Check sheet for the modelled part. Datum: model origin and axes. Units: mm. A direction names the side the tool comes from. Coordinates: 2 decimals unless noted, no trailing zeros. Loops run counter-clockwise (first coordinate to the right, second up) from the corner with the lowest first, then second, coordinate; pieces in that order, holes last. Notation, with made-up numbers: (30, -6.75) - (63, -6.75) arc R17 ccw to (63, 20.25) - close; hole circle Ø6 at (-8.75, 21). An arc over 180 degrees is marked (long way). Use a Markdown table: item, result. Add a question column.
1) Tool access check on faces 4 (the flat face through (4.144, 2.348, -9.615)), 5 (the flat face through (-4.11, 2.41, -22.75)), 6 (the flat face through (0, 4.762, -10)), 7 (the flat face through (7, 0, 26.683)), 8 (the cylindrical face through (-1.09, -4.91, 5.2)). Record the directions out of +Z, -Z, +X, -X, +Y, -Y that give a thin tool (end or side, any length) a straight path to the whole face; none if there is none.
2) Go/stop test with flat-tipped pins: P1, Ø3, axis at x = -5, y = -2, coming from the -Z side; P2, Ø4.5, axis at x = -0.5, z = -6, coming from the +Y side; P3, Ø3, axis at y = -3, z = -8.5, coming from the +X side; P4, Ø6, axis at x = 1, z = -21, coming from the -Y side. Record where each tip stops, or that it passes through.
3) Sectioned sample at A-A, the plane y = 5.75. Enter the section's corners in (x, z).
4) Sectioned sample at C-C, the plane z = 18. Enter the section's corners in (x, y).
5) Thickness scan on line 1 (Z direction, x = 2, y = -5.25); line 2 (Z direction, x = -3.5, y = -3); line 3 (Y direction, x = 1.75, z = -3). Record the ranges inside material, lowest first.
6) Draft check along Z on faces 1 (the flat face through (0, 0, 33.668)), 2 (the cylindrical face through (-0.834, 3.757, -18.219)), 3 (the flat face through (0, -6.375, 2)). Enter one of: pulls with the +Z half, pulls with the -Z half, needs draft (parallel to the pull), parting line crosses it, or undercut.
7) Sectioned sample at B-B, the plane z = -23.5. Enter the section's corners in (x, y), then the cut area to 3 significant figures.
Autodesk Inventor part; units mm, degrees
ref_plane "Work Plane1" through (0, 0, 15.2527) normal (0, 0, 1) x (1, 0, 0)
ref_plane "Work Plane2" through (0, 0, 5.7785) normal (0, 0, 1) x (1, 0, 0)
ref_plane "Work Plane3" through (0, 0, -18.7071) normal (0, 0, 1) x (1, 0, 0)
sketch "Sketch1" plane through (0, 0, 0) normal (0, 0, 1) x (1, 0, 0)
  line L0 (-10.3063, 0) -> (10.3063, 0)
  line L1 (0, -8.9256) -> (0, 8.9256)
  line L2 (3.6808, 6.3754) -> (7.3617, 0)
  line L3 (7.3617, 0) -> (3.6808, -6.3754)
  line L4 (3.6808, -6.3754) -> (-3.6808, -6.3754)
  line L5 (-3.6808, -6.3754) -> (-7.3617, 0)
  line L6 (-7.3617, 0) -> (-3.6808, 6.3754)
  line L7 (-3.6808, 6.3754) -> (3.6808, 6.3754)
  point P0 (0, 0)
  point P1 (0, 0)
  point P2 (0, 6.3754)
  dimension "d0" = 12.7508
extrude "Base" add sketch "Sketch1" along normal mid plane 67.3354
sketch "Sketch2" plane through (0, 0, 33.6677) normal (0, 0, 1) x (1, 0, 0)
  line L0 (7.3617, 0) -> (3.6808, -6.3754)
  line L1 (3.6808, 6.3754) -> (7.3617, 0)
  line L2 (-3.6808, 6.3754) -> (3.6808, 6.3754)
  line L3 (-7.3617, 0) -> (-3.6808, 6.3754)
  line L4 (-3.6808, -6.3754) -> (-7.3617, 0)
  line L5 (3.6808, -6.3754) -> (-3.6808, -6.3754)
  circle A0 centre (0, 0) radius 6.3754
extrude "Bearing Fit" cut sketch "Sketch2" against normal blind 6.985 contours L0 A0 L1 | L0 L5 A0 | A0 L2 L1 | L5 L4 A0 | A0 L3 L2 | L4 L3 A0
mirror "Mirror1" about plane through (0, 0, 0) normal (0, 0, 1) of "Bearing Fit"
sketch "Sketch4" plane through (0, 0, -33.6677) normal (0, 0, -1) x (-1, 0, 0)
  circle A0 centre (0, 0) radius 6.3754
  circle A1 centre (0, 0) radius 4.7625
  dimension "d7" = 9.525
extrude "Extrusion4" cut sketch "Sketch4" against normal up to surface (6.985 mm away)
sketch "Sketch5" plane through (3.6808, 6.3754, -26.6827) normal (0, 0, -1) x (-1, 0, 0)
  line L0 (7.3617, 0) -> (11.0425, -6.3754)
  line L1 (0, 0) -> (7.3617, 0)
  line L2 (-3.6808, -6.3754) -> (0, 0)
  line L3 (0, -12.7508) -> (-3.6808, -6.3754)
  line L4 (7.3617, -12.7508) -> (0, -12.7508)
  line L5 (11.0425, -6.3754) -> (7.3617, -12.7508)
  line L6 (6.4305, -1.6129) -> (9.1801, -6.3754)
  line L7 (9.1801, -6.3754) -> (6.4305, -11.1379)
  line L8 (6.4305, -11.1379) -> (0.9312, -11.1379)
  line L9 (0.9312, -11.1379) -> (-1.8184, -6.3754)
  line L10 (-1.8184, -6.3754) -> (0.9312, -1.6129)
  line L11 (0.9312, -1.6129) -> (6.4305, -1.6129)
  dimension "d10" = 9.525
extrude ".375 step down" cut sketch "Sketch5" against normal blind 25.4
ref_plane "Work Plane1" through (0, 0, 15.2527) normal (0, 0, 1) x (1, 0, 0)
sketch "Sketch6" plane through (0, 0, 15.2527) normal (0, 0, 1) x (1, 0, 0)
  line L0 (-3.6808, 6.3754) -> (0, 6.3754)
  line L1 (-5.5213, 3.1877) -> (-3.6808, 6.3754)
  line L2 (3.6808, 6.3754) -> (5.5213, 3.1877)
  line L3 (0, 6.3754) -> (3.6808, 6.3754)
  line L4 (5.5213, 3.1877) -> (7.3617, 0)
  line L5 (7.3617, 0) -> (5.5213, -3.1877)
  line L6 (5.5213, -3.1877) -> (3.6808, -6.3754)
  line L7 (0, -6.3754) -> (-3.6808, -6.3754)
  line L8 (-3.6808, -6.3754) -> (-5.5213, -3.1877)
  line L9 (3.6808, -6.3754) -> (0, -6.3754)
  line L10 (-7.3617, 0) -> (-5.5213, 3.1877)
  line L11 (-5.5213, -3.1877) -> (-7.3617, 0)
  circle A0 centre (0, 0) radius 5.0292
  point P0 (0, 0)
  dimension "d14" = 10.0584
extrude "Extrusion6" cut sketch "Sketch6" along normal blind 1.1684
ref_plane "Work Plane2" through (0, 0, 5.7785) normal (0, 0, 1) x (1, 0, 0)
sketch "Sketch7" plane through (0, 0, 5.7785) normal (0, 0, 1) x (1, 0, 0)
  line L0 (0, 6.3754) -> (3.6808, 6.3754)
  line L1 (3.6808, 6.3754) -> (5.5213, 3.1877)
  line L2 (5.5213, 3.1877) -> (7.3617, 0)
  line L3 (7.3617, 0) -> (5.5213, -3.1877)
  line L4 (5.5213, -3.1877) -> (3.6808, -6.3754)
  line L5 (3.6808, -6.3754) -> (0, -6.3754)
  line L6 (0, -6.3754) -> (-3.6808, -6.3754)
  line L7 (-3.6808, -6.3754) -> (-5.5213, -3.1877)
  line L8 (-7.3617, 0) -> (-5.5213, 3.1877)
  line L9 (-5.5213, 3.1877) -> (-3.6808, 6.3754)
  line L10 (-3.6808, 6.3754) -> (0, 6.3754)
  circle A0 centre (0, 0) radius 5.0292
  circle A1 centre (0, 0) radius 7.3617
  point P0 (0, 0)
  dimension "d18" = 10.0584
extrude "Extrusion7" cut sketch "Sketch7" against normal blind 1.1684
ref_plane "Work Plane3" through (0, 0, -18.7071) normal (0, 0, 1) x (1, 0, 0)
sketch "Sketch8" plane through (0, 0, -18.7071) normal (0, 0, 1) x (1, 0, 0)
  circle A0 centre (0, 0) radius 3.8481
  line L0 (-2.7496, 4.7625) -> (2.7496, 4.7625)
  line L1 (-5.4993, 0) -> (-2.7496, 4.7625)
  circle A1 centre (0, 0) radius 5.4993
  point P0 (0, 0)
  dimension "d22" = 7.6962
extrude "Extrusion8" cut sketch "Sketch8" along normal blind 0.9906
properties part number "shaft - step down No. 1 - 0.5 hex" material "Steel"
Solved:
| question | item | result |
|---|---|---|
| 1 | face 4 | -Z, +X, +Y |
| 1 | face 5 | -Z, -X, +Y |
| 1 | face 6 | -Z, +X, -X, +Y |
| 1 | face 7 | +Z, +X |
| 1 | face 8 | none |
| 2 | P1 | stops at z = -33.67 |
| 2 | P2 | stops at y = 4.76 |
| 2 | P3 | stops at x = 4.63 |
| 2 | P4 | stops at y = -4.76 |
| 3 | outline | (-4.04, -1.28) - (4.04, -1.28) - (4.04, 4.61) - (-4.04, 4.61) - close; (-4.04, 5.78) - (4.04, 5.78) - (4.04, 15.25) - (-4.04, 15.25) - close; (-4.04, 16.42) - (4.04, 16.42) - (4.04, 26.68) - (2.75, 26.68) - (2.75, 33.67) - (-2.75, 33.67) - (-2.75, 26.68) - (-4.04, 26.68) - close |
| 4 | outline | (-7.36, 0) - (-3.68, -6.38) - (3.68, -6.38) - (7.36, 0) - (3.68, 6.38) - (-3.68, 6.38) - close |
| 5 | line 1 | z = -1.28 to 4.61, 5.78 to 15.25, 16.42 to 33.67 |
| 5 | line 2 | z = -33.67 to -18.71, -17.72 to 33.67 |
| 5 | line 3 | y = -4.76 to 4.76 |
| 6 | face 1 | pulls with the +Z half |
| 6 | face 2 | undercut |
| 6 | face 3 | needs draft |
| 7 | outline | (-5.5, 0) - (-2.75, -4.76) - (2.75, -4.76) - (5.5, 0) - (2.75, 4.76) - (-2.75, 4.76) - close |
| 7 | area | 78.6 mm2 |
